Geometry check sheet. Reference: the model listing, model coordinates, mm. A direction names the side the tool comes from. Round coordinates to 2 decimals unless told otherwise and drop trailing zeros. Order: outer loops, then holes, each group sorted by start corner. A loop starts at its lowest first (then second) coordinate and runs counter-clockwise, first axis right, second up.
```python
from build123d import *

# Parameters (mm, degrees)
ESQUISSE1_W             = 33.75
ESQUISSE1_H             = 14
BOSS_EXTRU_1_DEPTH      = 1.9
ESQUISSE2_W             = 33.75
ESQUISSE2_H             = 30
ESQUISSE2_W_2           = 29.75
ESQUISSE2_H_2           = 26.1
BOSS_EXTRU_2_DEPTH      = 1.9
ENL_V_START             = -0.5
ESQUISSE4_W             = 31.75
ESQUISSE4_H             = 29
ENL_V_MAT_EXTRU_1_DEPTH = 0.5
CHANFREIN1_SIZE         = 0.3


with BuildPart() as part:
    # Esquisse1 → Boss.-Extru.1 (new body)
    with BuildSketch(Plane.XY):
        with Locations((16.875, 7)):
            Rectangle(ESQUISSE1_W, ESQUISSE1_H)
    extrude(amount=BOSS_EXTRU_1_DEPTH)

    # Esquisse2 → Boss.-Extru.2 (add)
    with BuildSketch(Plane(origin=(0, 14, 0), x_dir=(1, 0, 0), z_dir=(0, 1, 0))):
        with Locations((16.875, -15)):
            Rectangle(ESQUISSE2_W, ESQUISSE2_H)
        with Locations((16.875, -14.95)):
            Rectangle(ESQUISSE2_W_2, ESQUISSE2_H_2, mode=Mode.SUBTRACT)
    extrude(amount=BOSS_EXTRU_2_DEPTH)

    # Esquisse4 → Enlèv. mat.-Extru.1 (cut)
    with BuildSketch(Plane(origin=(0, 15.9, 0), x_dir=(1, 0, 0), z_dir=(0, 1, 0)).offset(ENL_V_START)):
        with Locations((16.875, -14.5)):
            Rectangle(ESQUISSE4_W, ESQUISSE4_H)
    extrude(amount=-ENL_V_MAT_EXTRU_1_DEPTH, mode=Mode.SUBTRACT)

    # Chanfrein1
    chanfrein1_edges = [part.edges().sort_by_distance(p)[0] for p in [
        (16.875, 14.9, 28),
        (16.875, 15.4, 0),
        (16.875, 14.9, 0),
        (1, 15.15, 0),
        (32.75, 15.15, 0),
        (16.875, 15.4, 28),
    ]]
    chamfer(chanfrein1_edges, length=CHANFREIN1_SIZE)


solid = part.part
```
(1) Sectioned sample at B-B, the plane z = 17.25. Record the cut outline in (x, y).
Returned:
outline: (0, 14) - (2, 14) - (2, 14.9) - (1, 14.9) - (1, 15.4) - (2, 15.4) - (2, 15.9) - (0, 15.9) - close; (31.75, 14) - (33.75, 14) - (33.75, 15.9) - (31.75, 15.9) - (31.75, 15.4) - (32.75, 15.4) - (32.75, 14.9) - (31.75, 14.9) - close
(2) Material ranges on line 1 (X direction, y = 14.25, z = 9.5); line 2 (Z direction, x = 16, y = 14.5); line 3 (Y direction, x = 32, z = 26.5), recorded low to high.
Returned:
line 1: x = 0 to 2, 31.75 to 33.75
line 2: z = 0 to 1.9, 28 to 30
line 3: y = 14 to 14.9, 15.4 to 15.9
(3) Set-up check for faces 1 (the flat face through (33.75, 14.4, 9.5)), 2 (the flat face through (16.8, 14, 28.4)): record each of +Z, -Z, +X, -X, +Y, -Y from which the full face is reachable in a straight line by a thin tool's end or side.
Returned:
face 1: +Z, -Z, +X, +Y, -Y
face 2: +Z, +X, -X, -Y
(4) Depth check by flat-ended pin: P1, Ø1, axis at y = 14.5, z = 11, coming from the -X side; P2, Ø4, axis at x = 4, y = 2.5, coming from the +Z side. Enter the tip coordinate at first touch or a pass-through.
Returned:
P1: stops at x = 0
P2: stops at z = 1.9
(5) Sectioned sample at C-C, the plane y = 9.75. Record the cut outline in (x, z).
Returned:
outline: (0, 0) - (33.75, 0) - (33.75, 1.9) - (0, 1.9) - close
(6) Draft check along X on faces 3 (the flat face through (2, 14.4, 15.3)), 4 (the flat face through (31.75, 14.4, 15.3)), 5 (the flat face through (17, 15, 30)), 6 (the flat face through (0, 14.4, 9.5)). Enter one of: released by +X, released by -X, zero draft, split by the parting line, or undercut.
Returned:
face 3: undercut
face 4: undercut
face 5: zero draft
face 6: released by -X
(7) Sectioned sample at A-A, the plane x = 13. Record the cut outline in (y, z), and give its area (3 significant figures).
Returned:
outline: (0, 0) - (14.6, 0) - (14.9, 0.3) - (14.9, 1.9) - (0, 1.9) - close; (14, 28) - (14.6, 28) - (14.9, 28.3) - (14.9, 29) - (15.4, 29) - (15.4, 28.3) - (15.7, 28) - (15.9, 28) - (15.9, 30) - (14, 30) - close; (15.4, 0.3) - (15.7, 0) - (15.9, 0) - (15.9, 1.9) - (15.4, 1.9) - close
area: 32.4 mm2
